Autodesk Inventor part; units mm, degrees
ref_plane "XY Plane" through (0, 0, 0) normal (0, 0, 1) x (1, 0, 0)
sketch "Skizze1" plane through (0, 0, 0) normal (0, 0, 1) x (1, 0, 0)
  circle A0 centre (0, 0) radius 31
  circle A1 centre (0, 0) radius 29
  dimension "d0" = 62
  dimension "d1" = 58
extrude "Extrusion1" add sketch "Skizze1" along normal mid plane 300
sketch "Skizze2" plane through (0, 0, 0) normal (0, 1, 0) x (-1, 0, 0)
  line L0 (-11, 169.5773) -> (-11, -169.8146) construction
  line L1 (-74.8376, 0) -> (82.6362, 0) construction
  line L2 (-11, 75) -> (-11, -75)
  line L3 (-31, -150) -> (-31, 150)
  line L4 (31, 150) -> (-31, 150)
  line L5 (-31, -150) -> (31, -150)
  spline S0 degree 2 poles (-11, 75) (-17.8298, 136.4739) (-72.8449, 128.3193) knots 0 0 0 1 1 1
  spline S1 degree 2 poles (-11, -75) (-17.6171, -136.2673) (-74.8376, -130) knots 0 0 0 1 1 1
  line L6 (-72.8449, 128.3193) -> (-74.8376, -130)
  line L7 (-31, 120) -> (-31, 150)
  line L8 (-31, 150) -> (31, 150)
  line L9 (31, 150) -> (31, -150)
  line L10 (31, -150) -> (31, 150)
  line L11 (31, -150) -> (-31, -150)
  line L12 (-31, -150) -> (-31, -120)
  point P0 (0, 0)
  dimension "d4" = 11
  dimension "d5" = 150
  dimension "d6" = 30
  dimension "d7" = 30
extrude "Extrusion3" cut sketch "Skizze2" along normal mid plane 100 contours S0 L3 L4 L9 L5 S1 L2
ref_plane "Arbeitsebene3" through (0, 33.25, 0) normal (0, 1, 0) x (-1, 0, 0)
sketch "Skizze8" plane through (0, 33.25, 0) normal (0, 1, 0) x (-1, 0, 0)
  line L0 (-11, -75) -> (-11, 75)
  arc A0 (-11, 56.4646) -> (-14.2842, 92.4804) centre (-300.1138, 48.2584) ccw
  arc A1 (-11, 56.4646) -> (-14.2842, 92.4804) centre (-31.6354, 72.7405) ccw
  point P0 (0, 0)
extrude "Extrusion6" cut sketch "Skizze8" against normal blind 65
mirror "Spiegeln2" about plane through (0, 0, 0) normal (0, 0, 1) of "Extrusion6"
ref_plane "Arbeitsebene7" through (15, 0, 0) normal (1, 0, 0) x (0, 1, 0)
sketch "Skizze16" plane through (15, 0, 0) normal (1, 0, 0) x (0, 1, 0)
  line L0 (80.6197, 79.5) -> (-53.6874, 79.5) construction
  line L1 (57.2311, 79.5) -> (-60.0661, 79.5)
  line L2 (-60.0661, 79.5) -> (-60.0661, 136.8193)
  line L3 (-60.0661, 136.8193) -> (57.2311, 136.8193)
  line L4 (57.2311, 136.8193) -> (57.2311, 79.5)
  point P0 (0, 0)
  point P1 (0, 120)
  dimension "d83" = 40.5
extrude "Extrusion15" cut sketch "Skizze16" against normal mid plane 35
ref_plane "Arbeitsebene8" through (27.75, 0, 0) normal (1, 0, 0) x (0, 1, 0)
sketch "Skizze17" plane through (27.75, 0, 0) normal (1, 0, 0) x (0, 1, 0)
  line L0 (0, 106.4673) -> (0, -19.1283) construction
  line L1 (26.1314, 79.5) -> (-26.1314, 79.5)
  line L2 (11, 79.5) -> (-11, 79.5)
  line L3 (-11, 79.5) -> (-11, 67.5)
  line L4 (-11, 67.5) -> (11, 67.5)
  line L5 (11, 67.5) -> (11, 79.5)
  point P0 (0, 0)
  dimension "d87" = 12
  dimension "d88" = 22
extrude "Extrusion16" add sketch "Skizze17" against normal blind 3
sketch "Skizze18" plane through (15, 0, 0) normal (1, 0, 0) x (0, 1, 0)
  line L0 (36.302, 52.5896) -> (-53.6938, 52.5896)
  line L1 (-53.6938, 52.5896) -> (-53.6938, -134.0275)
  line L2 (-53.6938, -134.0275) -> (36.302, -134.0275)
  line L3 (36.302, -134.0275) -> (36.302, 52.5896)
  point P0 (0, 0)
extrude "Extrusion17" cut sketch "Skizze18" along normal mid plane 35
properties part number "_3D-Druck"
Read the model definition and answer for the solid it produces. Units are mm, in the model's axes. A direction names the side the tool comes from. Give positions to 0.01 mm unless a question says otherwise; leave off trailing zeros. Order: outer loops, then holes, each group sorted by start corner. A loop starts at its lowest first (then second) coordinate and runs counter-clockwise, first axis right, second up.
(1) Find section B-B (y = -4). Give the vertices of the cut face in (x, z), plus the area to 3 significant figures.
(2) Find section D-D (y = -22). Give the vertices of the cut face in (x, z), plus the area to 3 significant figures.
(3) For faces 4 (the flat face through (24.75, 0, 74)), 5 (the cylindrical face through (30.996, 0.524, 65.856)), determine the directions among +Z, -Z, +X, -X, +Y, -Y from which every point of the face is accessible in a straight line to the end or side of a thin tool.
(4) Straight lines are drawn through the part: L1, parallel to X at y = 0, z = 74; L2, parallel to X at y = -11, z = 54.25; L3, parallel to Y at x = 19.25, z = 65.5. For each, find the intervals that lie inside material, in ascending order.
(5) For a pull along X with two mould halves and no side action, classify faces 1 (the flat face through (27.75, 0, 74)), 2 (the cylindrical face through (11.547, -27.537, 67.837)), 3 (the flat face through (26, 0, 67.5)) as released by +X, released by -X, zero draft, split by the parting line, or undercut.
(6) Given pin 1 (1.7 mm diameter, centred on x = 26, z = 71, fed in from +Y); pin 2 (6 mm diameter, centred on x = 25, z = 72.5, fed in from +Y); pin 3 (13 mm diameter, centred on y = 1.5, z = 71, fed in from +X); pin 4 (5 mm diameter, centred on x = 28.5, y = 0, fed in from +Z), each flat-ended and moving along its own axis, determine where each tip first touches the part or whether it passes through.
(7) Find section A-A (x = 16). Give the vertices of the cut face in (y, z).
(8) Find section C-C (z = 75.5). Give the vertices of the cut face in (x, y), plus the area to 3 significant figures.
Result sheet:
1. outline: (24.75, 67.5) - (27.75, 67.5) - (27.75, 79.5) - (24.75, 79.5) - close; (28.72, 52.59) - (30.74, 52.59) - (30.74, 79.5) - (28.72, 79.5) - close
1. area: 90.3 mm2
2. outline: (18.89, 52.59) - (21.84, 52.59) - (21.84, 79.5) - (18.89, 79.5) - close
2. area: 79.3 mm2
3. face 4: +Z, -Z, -X
3. face 5: +Z, -Z, +X
4. L1: x = 24.75 to 27.75, 29 to 31
4. L2: x = 26.83 to 28.98
4. L3: y = -24.3 to -21.69, 21.69 to 24.3
5. face 1: undercut
5. face 2: released by -X
5. face 3: zero draft
6. pin 1: stops at y = 18.12
6. pin 2: stops at y = 21.84
6. pin 3: stops at x = 31
6. pin 4: stops at z = 79.5
7. outline: (-26.55, 52.59) - (-24.19, 52.59) - (-24.19, 79.5) - (-26.55, 79.5) - close; (24.19, 52.59) - (26.55, 52.59) - (26.55, 79.5) - (24.19, 79.5) - close
8. outline: (12.17, -28.51) arc R31 ccw to (12.17, 28.51) - (12.17, 26.32) arc R29 cw to (26.83, 11) - (24.75, 11) - (24.75, -11) - (26.83, -11) arc R29 cw to (12.17, -26.32) - close; hole (27.75, -8.42) arc R29 ccw to (27.75, 8.42) - close
8. area: 202 mm2
